Geometry check sheet. Reference: the model listing, model coordinates, mm. Coordinates: 2 decimals unless noted, no trailing zeros. Order: outer loops, then holes, each group sorted by start corner. A loop starts at its lowest first (then second) coordinate and runs counter-clockwise, first axis right, second up. Notation, with made-up numbers: (10.25, 71.25) -> (33.25, 71.25) arc R13 cw to (33.25, 87.25) -> close; hole circle Ø9 at (7, 60.5). An arc over 180 degrees is marked (long way). Answer in a Markdown table with one row per item. Add a question column.
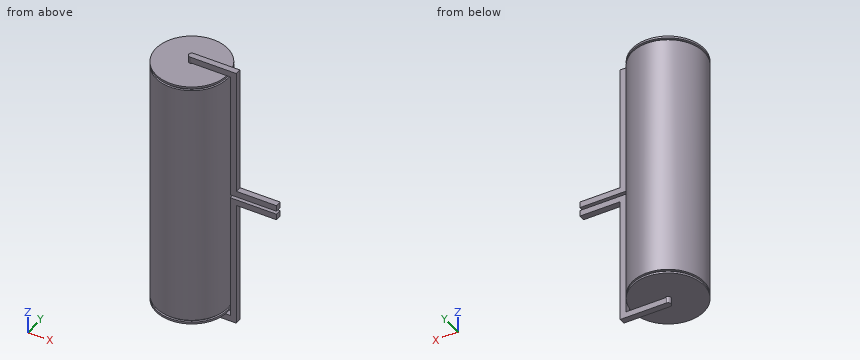
```python
from build123d import *

# Parameters (mm, degrees)
ESQUISSE1_R         = 9
BOSS_EXTRU_1_DEPTH  = 31
ESQUISSE3_R         = 8.5
BOSS_EXTRU_2_DEPTH  = 0.5
BOSS_EXTRU_3_START  = 0.5
ESQUISSE4_R         = 9
BOSS_EXTRU_3_DEPTH  = 0.5
ESQUISSE5_R         = 0.75
BOSS_EXTRU_4_DEPTH  = 0.2
BOSS_EXTRU_5_DEPTH  = 1.5
ESQUISSE7_W         = 1.5
ESQUISSE7_H         = 1.5
BOSS_EXTRU_6_DEPTH  = 31.8
ESQUISSE8_W         = 1.5
ESQUISSE8_H         = 1.5
BOSS_EXTRU_7_DEPTH  = 10
ESQUISSE10_R        = 9
BOSS_EXTRU_8_DEPTH  = 31
BOSS_EXTRU_9_START  = 0.5
ESQUISSE11_R        = 8.5
BOSS_EXTRU_9_DEPTH  = 0.5
ESQUISSE12_R        = 9
BOSS_EXTRU_10_DEPTH = 0.5
BOSS_EXTRU_11_START = 0.2
ESQUISSE13_R        = 0.75
BOSS_EXTRU_11_DEPTH = 0.2
BOSS_EXTRU_12_START = 1.5
BOSS_EXTRU_12_DEPTH = 1.5
ESQUISSE16_W        = 1.5
ESQUISSE16_H        = 1.5
BOSS_EXTRU_13_DEPTH = 31.8
ESQUISSE17_W        = 1.5
ESQUISSE17_H        = 1.5
BOSS_EXTRU_14_DEPTH = 10


with BuildPart() as part:
    # Esquisse1 → Boss.-Extru.1 (new body)
    with BuildSketch(Plane.XY):
        Circle(ESQUISSE1_R)
    extrude(amount=BOSS_EXTRU_1_DEPTH)

    # Esquisse3 → Boss.-Extru.2 (add)
    with BuildSketch(Plane(origin=(0, 0, 0), x_dir=(-1, 0, 0), z_dir=(0, 0, -1))):
        Circle(ESQUISSE3_R)
    extrude(amount=BOSS_EXTRU_2_DEPTH)

    # Esquisse4 → Boss.-Extru.3 (add)
    with BuildSketch(Plane(origin=(0, 0, -0.5), x_dir=(-1, 0, 0), z_dir=(0, 0, -1)).offset(BOSS_EXTRU_3_START)):
        with Locations(Location((0, 0, 0), (0, 0, 180))):
            Circle(ESQUISSE4_R)
    extrude(amount=-BOSS_EXTRU_3_DEPTH)

    # Esquisse5 → Boss.-Extru.4 (add)
    with BuildSketch(Plane(origin=(0, 0, -1), x_dir=(-1, 0, 0), z_dir=(0, 0, -1))):
        Circle(ESQUISSE5_R)
    extrude(amount=BOSS_EXTRU_4_DEPTH)

    # Esquisse6 → Boss.-Extru.5 (add)
    with BuildSketch(Plane(origin=(0, 0, -1.2), x_dir=(-1, 0, 0), z_dir=(0, 0, -1))):
        with BuildLine():
            Line((-11.5, -0.75), (0, -0.75))
            ThreePointArc((0, -0.75), (-0.75, 0), (0, 0.75))
            Line((0, 0.75), (-11.5, 0.75))
            Line((-11.5, 0.75), (-11.5, -0.75))
        make_face()
        with BuildLine():
            ThreePointArc((0, 0.75), (-0.75, 0), (0, -0.75))
            Line((0, -0.75), (0, 0.75))
        make_face()
        with BuildLine():
            Line((0, 0.75), (0, -0.75))
            ThreePointArc((0, -0.75), (0.530330086, -0.530330086), (0.75, 0))
            ThreePointArc((0.75, 0), (0.530330086, 0.530330086), (0, 0.75))
        make_face()
    extrude(amount=BOSS_EXTRU_5_DEPTH)

    # Esquisse7 → Boss.-Extru.6 (add)
    with BuildSketch(Plane.XY.offset(-1.2)):
        with Locations((10.75, 0)):
            Rectangle(ESQUISSE7_W, ESQUISSE7_H)
    extrude(amount=BOSS_EXTRU_6_DEPTH)

    # Esquisse8 → Boss.-Extru.7 (add)
    with BuildSketch(Plane(origin=(11.5, 0, 0), x_dir=(0, 0, -1), z_dir=(1, 0, 0))):
        with Locations((-29.85, 0)):
            Rectangle(ESQUISSE8_W, ESQUISSE8_H)
    extrude(amount=BOSS_EXTRU_7_DEPTH)

    # Esquisse10 → Boss.-Extru.8 (add)
    with BuildSketch(Plane.XY.offset(31)):
        Circle(ESQUISSE10_R)
    extrude(amount=BOSS_EXTRU_8_DEPTH)

    # Esquisse11 → Boss.-Extru.9 (add)
    with BuildSketch(Plane.XY.offset(62).offset(BOSS_EXTRU_9_START)):
        with Locations(Location((0, 0, 0), (0, 0, 180))):
            Circle(ESQUISSE11_R)
    extrude(amount=-BOSS_EXTRU_9_DEPTH)

    # Esquisse12 → Boss.-Extru.10 (add)
    with BuildSketch(Plane.XY.offset(62.5)):
        Circle(ESQUISSE12_R)
    extrude(amount=BOSS_EXTRU_10_DEPTH)

    # Esquisse13 → Boss.-Extru.11 (add)
    with BuildSketch(Plane.XY.offset(63).offset(BOSS_EXTRU_11_START)):
        with Locations(Location((0, 0, 0), (0, 0, 90))):
            Circle(ESQUISSE13_R)
    extrude(amount=-BOSS_EXTRU_11_DEPTH)

    # Esquisse15 → Boss.-Extru.12 (add)
    with BuildSketch(Plane.XY.offset(63.2).offset(BOSS_EXTRU_12_START)):
        with BuildLine():
            ThreePointArc((0.75, 0), (0.530330086, -0.530330086), (0, -0.75))
            Line((0, -0.75), (11.5, -0.75))
            Line((11.5, -0.75), (11.5, 0.75))
            Line((11.5, 0.75), (0, 0.75))
            ThreePointArc((0, 0.75), (0.530330086, 0.530330086), (0.75, 0))
        make_face()
        with BuildLine():
            ThreePointArc((0, 0.75), (-0.75, 0), (0, -0.75))
            Line((0, -0.75), (0, 0.75))
        make_face()
        with BuildLine():
            Line((0, 0.75), (0, -0.75))
            ThreePointArc((0, -0.75), (0.530330086, -0.530330086), (0.75, 0))
            ThreePointArc((0.75, 0), (0.530330086, 0.530330086), (0, 0.75))
        make_face()
    extrude(amount=-BOSS_EXTRU_12_DEPTH)

    # Esquisse16 → Boss.-Extru.13 (add)
    with BuildSketch(Plane(origin=(0, 0, 63.2), x_dir=(-1, 0, 0), z_dir=(0, 0, -1))):
        with Locations((-10.75, 0)):
            Rectangle(ESQUISSE16_W, ESQUISSE16_H)
    extrude(amount=BOSS_EXTRU_13_DEPTH)

    # Esquisse17 → Boss.-Extru.14 (add)
    with BuildSketch(Plane(origin=(11.5, 0, 0), x_dir=(0, 0, -1), z_dir=(1, 0, 0))):
        with Locations((-32.15, 0)):
            Rectangle(ESQUISSE17_W, ESQUISSE17_H)
    extrude(amount=BOSS_EXTRU_14_DEPTH)


solid = part.part
```
(1) Cross-section at B-B (x = 2.5). Enter the section's corners in (y, z), plus the area to 3 significant figures.
(2) Cross-section at A-A (z = 40.5). Enter the section's corners in (x, y).
(3) Cross-section at C-C (y = -6.5). Enter the section's corners in (x, z).
(4) Go/stop test with flat-tipped pins: P1, Ø8, axis at x = 16, y = 6, coming from the +Z side; P2, Ø12, axis at x = 9, z = 31.5, coming from the -Y side; P3, Ø5, axis at x = -2, z = 51, coming from the +Y side; P4, Ø0.8, axis at y = 0, z = 17.5, coming from the +X side. Record where each tip stops, or that it passes through.
(5) Cross-section at D-D (x = -1.5). Enter the section's corners in (y, z).
(6) Scan lines: line 1 along Z through (x, y) = (6.5, 0.5); line 2 along Y through (x, z) = (-3, 50.5); line 3 along Z through (x, y) = (7, -1). Record each from-to range of solid material in increasing order.
Checks:
| question | item | result |
|---|---|---|
| 1 | outline | (-8.65, -1) -> (8.65, -1) -> (8.65, -0.5) -> (8.12, -0.5) -> (8.12, 0) -> (8.65, 0) -> (8.65, 62) -> (8.12, 62) -> (8.12, 62.5) -> (8.65, 62.5) -> (8.65, 63) -> (-8.65, 63) -> (-8.65, 62.5) -> (-8.12, 62.5) -> (-8.12, 62) -> (-8.65, 62) -> (-8.65, 0) -> (-8.12, 0) -> (-8.12, -0.5) -> (-8.65, -0.5) -> close; (-0.75, -2.7) -> (0.75, -2.7) -> (0.75, -1.2) -> (-0.75, -1.2) -> close; (-0.75, 63.2) -> (0.75, 63.2) -> (0.75, 64.7) -> (-0.75, 64.7) -> close |
| 1 | area | 1,110 mm² |
| 2 | outline | circle Ø18 at (0, 0); (10, -0.75) -> (11.5, -0.75) -> (11.5, 0.75) -> (10, 0.75) -> close |
| 3 | outline | (-6.22, -1) -> (6.22, -1) -> (6.22, -0.5) -> (5.48, -0.5) -> (5.48, 0) -> (6.22, 0) -> (6.22, 62) -> (5.48, 62) -> (5.48, 62.5) -> (6.22, 62.5) -> (6.22, 63) -> (-6.22, 63) -> (-6.22, 62.5) -> (-5.48, 62.5) -> (-5.48, 62) -> (-6.22, 62) -> (-6.22, 0) -> (-5.48, 0) -> (-5.48, -0.5) -> (-6.22, -0.5) -> close |
| 4 | P1 | through |
| 4 | P2 | y = -8.49 |
| 4 | P3 | y = 9 |
| 4 | P4 | x = 11.5 |
| 5 | outline | (-8.87, -1) -> (8.87, -1) -> (8.87, -0.5) -> (8.37, -0.5) -> (8.37, 0) -> (8.87, 0) -> (8.87, 62) -> (8.37, 62) -> (8.37, 62.5) -> (8.87, 62.5) -> (8.87, 63) -> (-8.87, 63) -> (-8.87, 62.5) -> (-8.37, 62.5) -> (-8.37, 62) -> (-8.87, 62) -> (-8.87, 0) -> (-8.37, 0) -> (-8.37, -0.5) -> (-8.87, -0.5) -> close |
| 6 | line 1 | -2.7 to -1.2, -1 to 63, 63.2 to 64.7 |
| 6 | line 2 | -8.49 to 8.49 |
| 6 | line 3 | -1 to 63 |
